Here's how the part is built. I have some questions about the finished solid (model axes, mm). Face numbers are marked on the shaded views. A direction names the side the tool comes from. Coordinates: 2 decimals unless noted, no trailing zeros. Write each loop counter-clockwise with the first axis right and the second up, starting at its lowest first coordinate (ties: lowest second). Pieces come first, ordered by that corner, then holes.
(1) Thinking about a two-plate mould opening in Y: for the marked faces 1, 2, 3 and 4, which applies, released by +Y, released by -Y, zero draft, split by the parting line, or undercut?
(2) Please list where these lines run through material, in increasing order: probe 1 along X at (y, z) = (5.5, -13.25); probe 2 along Z at (x, y) = (5.25, 11.25); probe 3 along X at (y, z) = (7, -2.75).
(3) For pin 1 Ø1.2 at (y, z) = (8.5, -7.5) entering from -X; pin 2 Ø5 at (y, z) = (0, -3.5) entering from -X; pin 3 Ø1.6 at (y, z) = (8.5, -9) entering from +X, each with a flat end and sliding along its axis, tell me the tip position at first contact or that it passes through.
(4) Which directions (+Z, -Z, +X, -X, +Y, -Y) give clear straight access to the entire face, cutting with the end or side of a thin tool? Please do the marked faces 5 and 6.
(5) Imagine slicing it at A-A, the plane z = -10.25. State how many separate pieces and enclosed holes the cut face has, plus the area to 3 significant figures.
(6) Imagine slicing it at B-B, the plane z = 1.25. List the corners of the cut face in (x, y) for me.
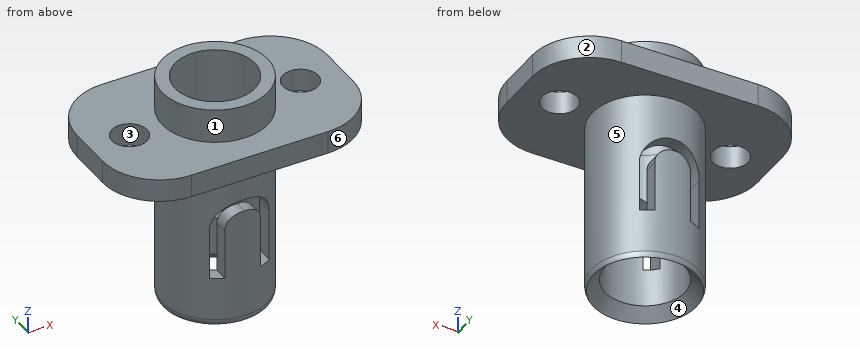
```python
from build123d import *

# Parameters (mm, degrees)
ESQUISSE1_W               = 22
ESQUISSE1_H               = 14
BOSS_EXTRU_1_DEPTH        = 2
ESQUISSE3_R               = 4.625
ESQUISSE3_R_2             = 3.5
BOSS_EXTRU_2_DEPTH        = 15
BOSS_EXTRU_3_START        = 3
ESQUISSE5_R               = 4.625
BOSS_EXTRU_3_DEPTH        = 3
ESQUISSE4_R               = 3.5
ENL_V_MAT_EXTRU_1_DEPTH   = 24.243966888
ENL_V_MAT_EXTRU_2_DEPTH   = 21.826081473
CONG_1_R                  = 5
D_GAGEMENT_M2_51_D        = 3.1
D_GAGEMENT_M2_51_DEPTH    = 18.17
D_GAGEMENT_M2_51_TIP      = 0.931333959
CHANFREIN1_SIZE           = 1
CONG_2_R                  = 1
ESQUISSE12_R              = 1.5
BOSS_EXTRU_4_DEPTH        = 1.35
BOSS_EXTRU_4_DRAFT        = -32
SYM_TRIE2_COPY_1_SKETCH_R = 1.5
SYM_TRIE2_COPY_1_DEPTH    = 1.35
SYM_TRIE2_COPY_1_DRAFT    = -32


with BuildPart() as part:
    # Esquisse1 → Boss.-Extru.1 (new body)
    with BuildSketch(Plane.XY):
        with Locations((-1.638262124, 5.472222222)):
            Rectangle(ESQUISSE1_W, ESQUISSE1_H)
    extrude(amount=BOSS_EXTRU_1_DEPTH)

    # Esquisse3 → Boss.-Extru.2 (add)
    with BuildSketch(Plane(origin=(0, 0, 0), x_dir=(-1, 0, 0), z_dir=(0, 0, -1))):
        with Locations(Location((1.638262124, 5.472222222, 0), (0, 0, 180))):
            Circle(ESQUISSE3_R)
        with Locations((1.638262124, 5.472222222)):
            Circle(ESQUISSE3_R_2, mode=Mode.SUBTRACT)
    extrude(amount=BOSS_EXTRU_2_DEPTH)

    # Esquisse5 → Boss.-Extru.3 (add)
    with BuildSketch(Plane.XY.offset(2).offset(BOSS_EXTRU_3_START)):
        with Locations((-1.638262124, 5.472222222)):
            Circle(ESQUISSE5_R)
    extrude(amount=-BOSS_EXTRU_3_DEPTH)

    # Esquisse4 → Enlèv. mat.-Extru.1 (cut, through all)
    with BuildSketch(Plane(origin=(0, 0, 0), x_dir=(-1, 0, 0), z_dir=(0, 0, -1))):
        with Locations((1.638262124, 5.472222222)):
            Circle(ESQUISSE4_R)
    extrude(amount=-ENL_V_MAT_EXTRU_1_DEPTH, mode=Mode.SUBTRACT)

    # Esquisse6 → Enlèv. mat.-Extru.2 (cut, symmetric)
    with BuildSketch(Plane(origin=(0, 5.472222222, 0), x_dir=(-1, 0, 0), z_dir=(0, -1, 0))):
        with BuildLine():
            Line((3.21697524, 10.683041), (4.265016312, 10.683041))
            Line((4.265016312, 10.683041), (4.265016312, 6.204978645))
            ThreePointArc((4.265016312, 6.204978645), (3.485411067, 4.403002531), (1.638262124, 3.737462868))
            Line((1.638262124, 3.737462868), (1.638262124, 4.790102764))
            ThreePointArc((1.638262124, 4.790102764), (2.74581304, 5.165435363), (3.21697524, 6.235738952))
            Line((3.21697524, 6.235738952), (3.21697524, 10.683041))
        make_face()
    enl_v_mat_extru_2 = extrude(amount=ENL_V_MAT_EXTRU_2_DEPTH, both=True, mode=Mode.SUBTRACT)

    # Symétrie1: Enlèv. mat.-Extru.2 across plane
    add(enl_v_mat_extru_2.mirror(Plane.ZY.offset(1.638262124)), mode=Mode.SUBTRACT)

    # Congé1
    cong_1_edges = [part.edges().sort_by_distance(p)[0] for p in [
        (-12.638262124, 12.472222222, 1),
        (9.361737876, 12.472222222, 1),
        (9.361737876, -1.527777778, 1),
        (-12.638262124, -1.527777778, 1),
    ]]
    fillet(cong_1_edges, radius=CONG_1_R)

    # Dégagement M2.51
    with Locations(Plane(origin=(0, 0, 0), x_dir=(-1, 0, 0), z_dir=(0, 0, -1))):
        with Locations((-5.861737876, 5.472222222), (9.138262124, 5.472222222)):
            Hole(D_GAGEMENT_M2_51_D / 2, depth=D_GAGEMENT_M2_51_DEPTH)
            with Locations((0, 0, -(D_GAGEMENT_M2_51_DEPTH + D_GAGEMENT_M2_51_TIP / 2))):  # 118° drill point
                Cone(0, D_GAGEMENT_M2_51_D / 2, D_GAGEMENT_M2_51_TIP, mode=Mode.SUBTRACT)

    # Chanfrein1
    chanfrein1_edges = [part.edges().sort_by_distance(p)[0] for p in [
        (1.861737876, 5.472222222, -15),
    ]]
    chamfer(chanfrein1_edges, length=CHANFREIN1_SIZE)

    # Congé2
    # the kernel refuses this fillet: 1 mm, written as the material it takes off along each edge
    with BuildSketch(Plane(origin=(-1.638262124, 5.472222222, -15), x_dir=(1, 0, 0), z_dir=(0, 1, 0))) as cong_2_piece_1:
        with BuildLine():
            CenterArc((3.625, -0.484122918), CONG_2_R, 0, 28.955024372)
            Line((4.625, -0.484122918), (4.645, -0.484122918))
            Line((4.645, -0.484122918), (4.645, 0))
            Line((4.645, 0), (4.625, 0.02))
            ThreePointArc((4.625, 0.02), (4.5625, 0.02), (4.5175, 0.009682458))
            Line((4.5175, 0.009682458), (4.5, 0))
        make_face()
    revolve(axis=Axis((-1.638262124, 5.472222222, -15), (0, 0, -1)), mode=Mode.SUBTRACT)


with BuildPart() as boss_extru_4_tool:
    # Esquisse12 → Boss.-Extru.4 (with draft: the straight prism first)
    with BuildSketch(Plane(origin=(0, 1.972222222, 0), x_dir=(-1, 0, 0), z_dir=(0, -1, 0))):
        with Locations((1.626150822, 6.5)):
            Circle(ESQUISSE12_R)
    extrude(amount=-BOSS_EXTRU_4_DEPTH)
    # Boss.-Extru.4: the draft: its side faces are tilted about the plane it starts from
    boss_extru_4_sides = [boss_extru_4_tool.faces().sort_by_distance(p)[0] for p in [
        (-0.126150822, 2.647222222, -6.5),
    ]]
    draft(boss_extru_4_sides, Plane(origin=(0, 1.972222222, 0), x_dir=(-1, 0, 0), z_dir=(0, -1, 0)), BOSS_EXTRU_4_DRAFT)


with BuildPart() as part_1:
    add(part.part)

    # Boss.-Extru.4: add boss_extru_4_tool
    add(boss_extru_4_tool.part)


with BuildPart() as sym_trie2_copy_1_tool:
    # Symétrie2 copy 1 sketch → Symétrie2 copy 1 (with draft: the straight prism first)
    with BuildSketch(Plane(origin=(0, 8.972222222, 0), x_dir=(-1, 0, 0), z_dir=(0, 1, 0))):
        with Locations((1.626150822, -6.5)):
            Circle(SYM_TRIE2_COPY_1_SKETCH_R)
    extrude(amount=-SYM_TRIE2_COPY_1_DEPTH)
    # Symétrie2 copy 1: the draft: its side faces are tilted about the plane it starts from
    sym_trie2_copy_1_sides = [sym_trie2_copy_1_tool.faces().sort_by_distance(p)[0] for p in [
        (-0.126150822, 8.297222222, -6.5),
    ]]
    draft(sym_trie2_copy_1_sides, Plane(origin=(0, 8.972222222, 0), x_dir=(-1, 0, 0), z_dir=(0, 1, 0)), SYM_TRIE2_COPY_1_DRAFT)


with BuildPart() as part_2:
    add(part_1.part)

    # Symétrie2 copy 1: add sym_trie2_copy_1_tool
    add(sym_trie2_copy_1_tool.part)


solid = part_2.part
```
Recorded:
1. face 1: split by the parting line
1. face 2: released by +Y
1. face 3: undercut
1. face 4: undercut
2. probe 1: x = -6.26 to -5.14, 1.86 to 2.99
2. probe 2: z = 0 to 2
2. probe 3: x = -6 to -4.79, 1.51 to 2.73
3. pin 1: stops at x = -5.57
3. pin 2: stops at x = -5.18
3. pin 3: stops at x = 2.41
4. face 5: -Z
4. face 6: +Z, -Z, +X, -Y
5. separate pieces: 4
5. enclosed holes: 0
5. area: 23.1 mm2
6. outline: (-12.64, 3.47) arc R5 ccw to (-7.64, -1.53) - (4.36, -1.53) arc R5 ccw to (9.36, 3.47) - (9.36, 7.47) arc R5 ccw to (4.36, 12.47) - (-7.64, 12.47) arc R5 ccw to (-12.64, 7.47) - close; hole circle Ø3.1 at (-9.14, 5.47); hole circle Ø7 at (-1.64, 5.47); hole circle Ø3.1 at (5.86, 5.47)
